Here's the drawing with two shaded views (mm, measured from the low corner). I have some questions. A direction names the side the tool comes from. Coordinates: 2 decimals unless noted, no trailing zeros. Write each loop counter-clockwise with the first axis right and the second up, starting at its lowest first coordinate (ties: lowest second). Pieces come first, ordered by that corner, then holes.
Item 1: For P1, Ø12, axis at x = 14.5, z = 67, coming from the -Y side; P2, Ø1, axis at x = 8, z = 142, coming from the -Y side; P3, Ø1, axis at x = 9, y = 4, coming from the +Z side, each with a flat end and sliding along its axis, tell me the tip position at first contact or that it passes through.
Item 2: If I drill on probe 1 along Y at (x, z) = (14.5, 16); probe 2 along Z at (x, y) = (9.25, 5.5); probe 3 along X at (y, z) = (14.75, 217.5), over which ranges is the centre line in solid material (lowest first)?
Item 3: I want a section at B-B on x = 2.75. Please give me the cut outline in (y, z), then the cut area to 3 significant figures.
Item 4: Which directions (+Z, -Z, +X, -X, +Y, -Y) give clear straight access to the entire face, cutting with the end or side of a thin tool? Please do the marked faces 1 and 2.
Item 5: I want a section at A-A on z = 247. Please give me the cut outline in (x, y).
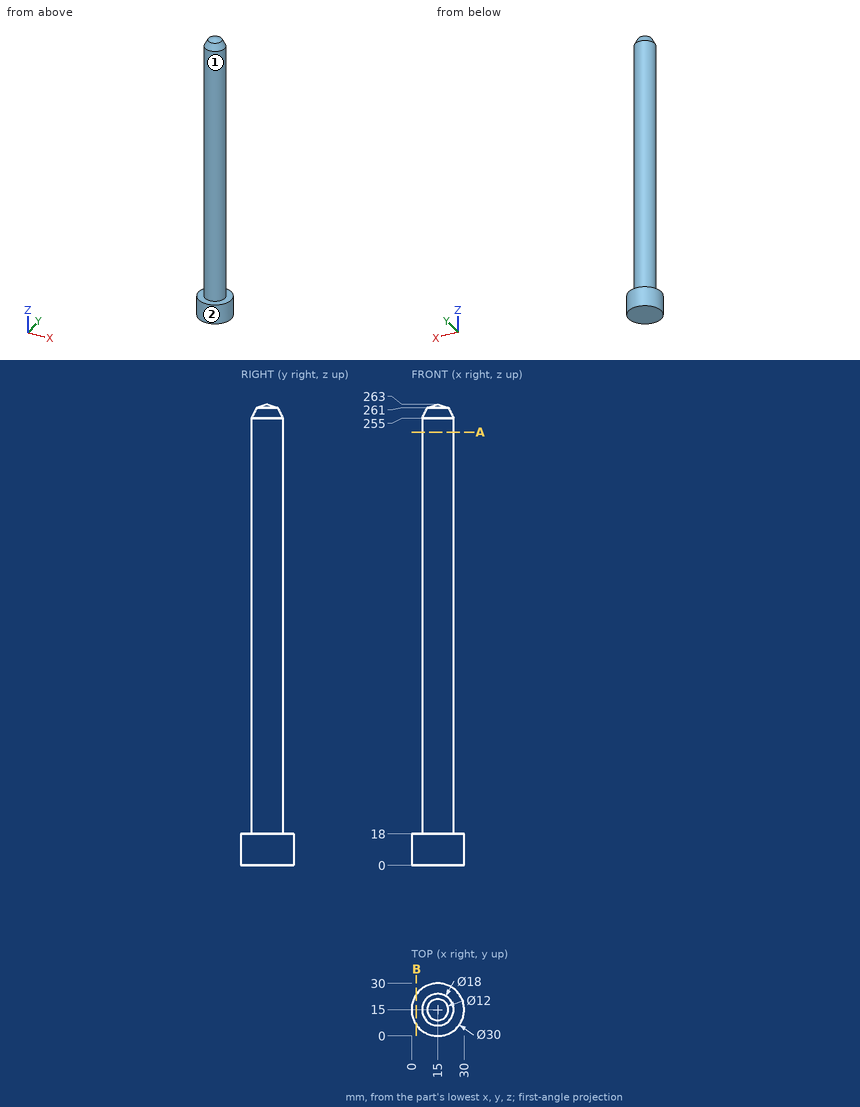
Response values:
1. P1: stops at y = 6
1. P2: stops at y = 8.78
1. P3: stops at z = 18
2. probe 1: y = 0.01 to 29.99
2. probe 2: z = 0 to 18
2. probe 3: x = 6 to 24
3. outline: (6.34, 0) - (23.66, 0) - (23.66, 18) - (6.34, 18) - close
3. area: 312 mm2
4. face 1: +Z
4. face 2: +Z, -Z
5. outline: circle Ø18 at (15, 15)
